Source: three-view drawing plus pictorial views. Frame: mm from the lowest corner of the part. A direction names the side the tool comes from. Give positions to 0.01 mm unless a question says otherwise; leave off trailing zeros. Loops run counter-clockwise (first coordinate to the right, second up) from the corner with the lowest first, then second, coordinate; pieces in that order, holes last. Notation, with made-up numbers: (10.25, -27.5) - (19.25, -27.5) arc R27 ccw to (19.25, -10.5) - close; hole circle Ø5 at (13, 5). An arc over 180 degrees is marked (long way). Answer as a JSON object with one key per item and string values. Group by question number.
(1) Section query A-A (y = 25). Return loops of the section in (x, z).
(2) Section query C-C (x = 22.5). Return loops of the section in (y, z).
(3) Pin query (flat end, axial travel): P1, Ø25, axis at y = 28.5, z = 20.5, coming from the +X side; P2, Ø20, axis at x = 23, y = 19, coming from the -Z side. Return the tip coordinate at first contact, or that it passes through.
(4) Section query B-B (z = 52.5). Return loops of the section in (x, y), plus the area to 3 significant figures.
(5) Access query for the marked faces 4, 5 and 6. Directions: +Z, -Z, +X, -X, +Y, -Y. A direction counts if a zero-diameter tool reaches every point of the face in a straight line with its end or side. Return the directions, or none.
(6) Section query D-D (z = 31.5). Return loops of the section in (x, y).
(7) Material intervals for L1, parallel to X at y = 11.5, z = 27.5; L2, parallel to Z at x = 5, y = 25; L3, parallel to X at y = 44, z = 4, sorted ascending.
(8) Mould query, pull axis Z, two halves, no side actions, for the marked faces 1, 2 and 3. Classes: +Z half, -Z half, draft (parallel to the pull), parting line (faces both ways), or undercut.
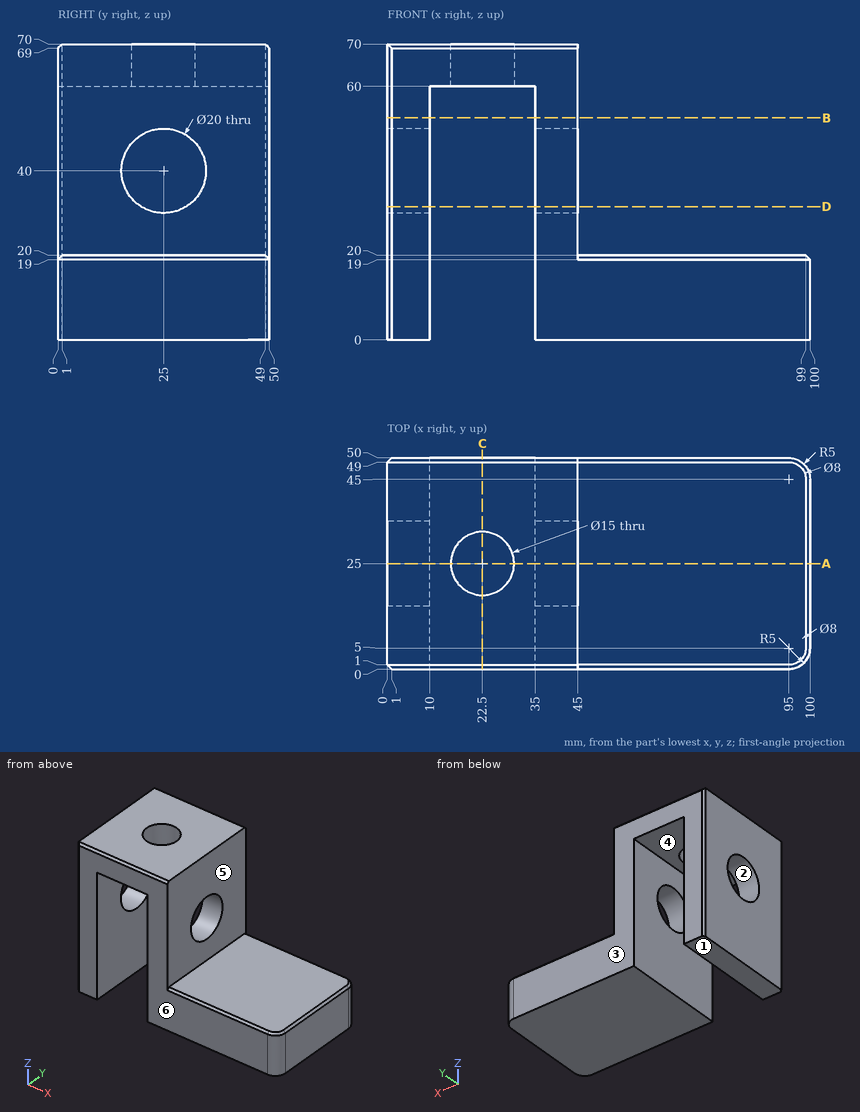
Recorded:
{
 "1": {"outline": "(0, 0) - (10, 0) - (10, 30) - (0, 30) - close; (0, 50) - (10, 50) - (10, 60) - (15, 60) - (15, 70) - (0, 70) - close; (30, 60) - (35, 60) - (35, 50) - (45, 50) - (45, 70) - (30, 70) - close; (35, 0) - (100, 0) - (100, 19) - (99, 20) - (45, 20) - (45, 30) - (35, 30) - close"},
 "2": {"outline": "(0, 60) - (17.5, 60) - (17.5, 70) - (1, 70) - (0, 69) - close; (32.5, 60) - (50, 60) - (50, 69) - (49, 70) - (32.5, 70) - close"},
 "3": {"P1": "stops at x = 100", "P2": "stops at z = 60"},
 "4": {"outline": "(0, 1) - (1, 0) - (10, 0) - (10, 50) - (1, 50) - (0, 49) - close; (35, 0) - (45, 0) - (45, 50) - (35, 50) - close", "area": "999 mm^2"},
 "5": {"face 4": "-Z, +Y, -Y", "face 5": "+Z, +X, +Y, -Y", "face 6": "+Z, -Z, +X, -X, -Y"},
 "6": {"outline": "(0, 1) - (1, 0) - (10, 0) - (10, 19.73) - (0, 19.73) - close; (0, 30.27) - (10, 30.27) - (10, 50) - (1, 50) - (0, 49) - close; (35, 0) - (45, 0) - (45, 19.73) - (35, 19.73) - close; (35, 30.27) - (45, 30.27) - (45, 50) - (35, 50) - close"},
 "7": {"L1": "x = 0 to 10, 35 to 45", "L2": "z = 0 to 30, 50 to 70", "L3": "x = 0 to 10, 35 to 100"},
 "8": {"face 1": "-Z half", "face 2": "undercut", "face 3": "draft"}
}
